from build123d import *

# Parameters (mm, degrees)
SKETCH1_R               = 14.2875
BOSS_EXTRUDE1_DEPTH     = 16.383
SKETCH2_R               = 6.35
BOSS_EXTRUDE2_DEPTH     = 6.35
SKETCH4_R               = 1.1811
CUT_EXTRUDE1_DEPTH      = 23.733
CHAMFER1_SIZE           = 0.508
CUT_EXTRUDE2_DEPTH      = 18.923
CUT_REVOLVE1_ANGLE      = 5
SKETCH7_R               = 0.635
F_1_4_20_TAPPED_HOLE1_D = 5.1054
HOLE1_D                 = 8.128
HOLE1_DEPTH             = 5.08
CHAMFER2_SIZE           = 0.254


with BuildPart() as part:
    # Sketch1 → Boss-Extrude1 (new body)
    with BuildSketch(Plane(origin=(0, 0, 0), x_dir=(1, 0, 0), z_dir=(0, 1, 0))):
        with Locations(Location((0, 0, 0), (0, 0, 270))):  # turned: the seam where the file's is
            Circle(SKETCH1_R)
    extrude(amount=BOSS_EXTRUDE1_DEPTH)

    # Sketch2 → Boss-Extrude2 (add)
    with BuildSketch(Plane.XZ):
        with Locations(Location((0, 0, 0), (0, 0, 90))):  # turned: the seam where the file's is
            Circle(SKETCH2_R)
    extrude(amount=BOSS_EXTRUDE2_DEPTH)

    # Sketch4 → Cut-Extrude1 (cut, through all)
    with BuildSketch(Plane(origin=(0, 16.383, 0), x_dir=(1, 0, 0), z_dir=(0, 1, 0))):
        with Locations(Location((0, 10.16, 0), (0, 0, 270))):  # turned: the seam where the file's is
            Circle(SKETCH4_R)
    extrude(amount=-CUT_EXTRUDE1_DEPTH, mode=Mode.SUBTRACT)

    # Chamfer1
    chamfer1_edges = [part.edges().sort_by_distance(p)[0] for p in [
        (0, 0, -14.2875),
        (0, 16.383, -14.2875),
        (0, -6.35, -6.35),
    ]]
    chamfer(chamfer1_edges, length=CHAMFER1_SIZE)

    # Sketch5 → Cut-Extrude2 (cut, symmetric)
    with BuildSketch(Plane.XY):
        Polygon((-2.548384182, 18.669), (-16.088719044, 5.128665138), (-16.088719044, 23.827435377), (16.088719044, 23.827435377), (16.088719044, 5.128665138), (2.548384182, 18.669), align=None)
    extrude(amount=CUT_EXTRUDE2_DEPTH, both=True, mode=Mode.SUBTRACT)

    # Sketch6 → Cut-Revolve1 (revolve, symmetric, cut)
    with BuildSketch(Plane.XY) as cut_revolve1_sk:
        with BuildLine():
            Line((0.60449584, 21.537658497), (-20.777423288, 21.537658497))
            Line((-20.777423288, 21.537658497), (-20.777423288, 0.072260804))
            ThreePointArc((-20.777423288, 0.072260804), (-10.249089347, 10.966952825), (0.60449584, 21.537658497))
        make_face()
    cut_revolve1 = revolve(axis=Axis((343.991741396, -341.896241396, 0), (0, 1, 0)), revolution_arc=CUT_REVOLVE1_ANGLE / 2, mode=Mode.SUBTRACT)
    cut_revolve1 = cut_revolve1 + revolve(cut_revolve1_sk.sketch, axis=Axis((343.991741396, -341.896241396, 0), (0, -1, 0)), revolution_arc=CUT_REVOLVE1_ANGLE / 2, mode=Mode.SUBTRACT)

    # Mirror1: Cut-Revolve1 across plane
    add(cut_revolve1.mirror(Plane(origin=(0, 0, 0), x_dir=(0, 0, 1), z_dir=(1, 0, 0))), mode=Mode.SUBTRACT)

    # Sketch7 → Cut-Revolve2 (revolve, cut)
    with BuildSketch(Plane.XY, mode=Mode.PRIVATE) as cut_revolve2_sk:
        with Locations((6.799012806, -0.449012806)):
            Circle(SKETCH7_R)
    revolve(cut_revolve2_sk.sketch.rotate(Axis((0, 16.383, 0), (0, -1, 0)), 90), axis=Axis((0, 16.383, 0), (0, -1, 0)), mode=Mode.SUBTRACT)  # turned: the seam where the file's is

    # 1/4-20 Tapped Hole1 (through all)
    with Locations(Plane(origin=(0, 16.383, 0), x_dir=(1, 0, 0), z_dir=(0, 1, 0))):
        with Locations((0, 0)):
            Hole(F_1_4_20_TAPPED_HOLE1_D / 2)

    # Hole1
    with Locations(Plane(origin=(0, 16.383, 0), x_dir=(1, 0, 0), z_dir=(0, 1, 0))):
        with Locations((0, 0)):
            Hole(HOLE1_D / 2, depth=HOLE1_DEPTH)

    # Chamfer2
    chamfer2_edges = [part.edges().sort_by_distance(p)[0] for p in [
        (2.5527, -6.35, 0),
        (2.5527, 11.303, 0),
        (4.064, 16.383, 0),
    ]]
    chamfer(chamfer2_edges, length=CHAMFER2_SIZE)


solid = part.part
Could you check a few things on this model? Use its own coordinates, in mm. A direction names the side the tool comes from. Give positions to 0.01 mm unless a question says otherwise; leave off trailing zeros. Order: outer loops, then holes, each group sorted by start corner. A loop starts at its lowest first (then second) coordinate and runs counter-clockwise, first axis right, second up. Notation, with made-up numbers: (-11.75, 25.5) -> (29.25, 25.5) arc R9 cw to (29.25, 32.5) -> close; hole circle Ø7 at (-30.5, -35.75). An arc over 180 degrees is marked (long way). Answer in a Markdown table with one row per item. Add a question column.
Item 1: For faces 4 (the flat face through (3.2, 16.383, -3.3)), 5 (the cylindrical face through (3.86, -3.34, -5.04)), 6 (the flat face through (1, 11.303, 3)), which set-ups out of +Z, -Z, +X, -X, +Y, -Y let a thin tool reach every point of the face, with its end or its side?
Item 2: Please list where these lines run through material, in increasing order: probe 1 along X at (y, z) = (3.25, 0); probe 2 along X at (y, z) = (12.6, 0); probe 3 along Z at (x, y) = (-1, -5.5).
Item 3: I'm going to push flat-ended pins straight in: P1, Ø6.5, axis at x = -0.5, z = 0.5, coming from the +Y side; P2, Ø6, axis at y = -2.5, z = 2, coming from the +X side; P3, Ø10, axis at x = 8, y = 9, coming from the -Z side; P4, Ø1.9, axis at x = 0, z = -10.16, coming from the -Y side. Where does each tip first touch, or does it pass through?
Item 4: We'd pull the mould along X, two halves only. Please class faces 1 (the cylindrical face through (0.881, 13.682, 3.967)), 2 (the conical face through (-0.07, 16.245, 13.917)), 3 (the flat face through (-6, 0, 6)): pulls with the +X half, pulls with the -X half, needs draft (parallel to the pull), parting line crosses it, or undercut.
Item 5: Imagine slicing it at A-A (x = 0). Count the separate pieces of the cut face and the enclosed holes in it, and give its area (3 significant figures).
Item 6: Imagine slicing it at C-C (y = 3.5). List the corners of the cut face in (x, z) for me (1 decimal), and give its area (3 significant figures).
Item 7: Imagine slicing it at B-B (y = -2.5). List the corners of the cut face in (x, z) for me, and give its area (3 significant figures).
Result:
| question | item | result |
|---|---|---|
| 1 | face 4 | +Z, -Z, +X, -X, +Y |
| 1 | face 5 | -Y |
| 1 | face 6 | +Y |
| 2 | probe 1 | -14.29 to -2.55, 2.55 to 14.29 |
| 2 | probe 2 | -8.61 to -4.06, 4.06 to 8.61 |
| 2 | probe 3 | -6.27 to -2.35, 2.35 to 6.27 |
| 3 | P1 | y = 11.3 |
| 3 | P2 | x = 14.16 |
| 3 | P3 | z = -13.97 |
| 3 | P4 | through |
| 4 | face 1 | undercut |
| 4 | face 2 | parting line crosses it |
| 4 | face 3 | needs draft |
| 5 | separate pieces | 3 |
| 5 | enclosed holes | 0 |
| 5 | area | 377 mm2 |
| 6 | outline | circle Ø28.6 at (0, 0); hole circle Ø5.1 at (0, 0); hole circle Ø2.4 at (0, -10.2) |
| 6 | area | 616 mm2 |
| 7 | outline | circle Ø12.7 at (0, 0); hole circle Ø5.11 at (0, 0) |
| 7 | area | 106 mm2 |
